```python
from build123d import *

# Parameters (mm, degrees)
SKETCH2_W           = 9.5
SKETCH2_H           = 9.5
BOSS_EXTRUDE1_DEPTH = 5
SKETCH3_R           = 4
BOSS_EXTRUDE2_DEPTH = 4
SKETCH4_R           = 3.25
BOSS_EXTRUDE3_DEPTH = 1.5
BOSS_EXTRUDE4_DEPTH = 7


with BuildPart() as part:
    # Sketch2 → Boss-Extrude1 (new body)
    with BuildSketch(Plane(origin=(0, 0, 0), x_dir=(1, 0, 0), z_dir=(0, 1, 0))):
        Rectangle(SKETCH2_W, SKETCH2_H)
    extrude(amount=BOSS_EXTRUDE1_DEPTH)

    # Sketch3 → Boss-Extrude2 (add)
    with BuildSketch(Plane(origin=(0, 5, 0), x_dir=(1, 0, 0), z_dir=(0, 1, 0))):
        with Locations(Location((0, 0, 0), (0, 0, 270))):
            Circle(SKETCH3_R)
    extrude(amount=BOSS_EXTRUDE2_DEPTH)

    # Sketch4 → Boss-Extrude3 (add)
    with BuildSketch(Plane(origin=(0, 9, 0), x_dir=(1, 0, 0), z_dir=(0, 1, 0))):
        with Locations(Location((0, 0, 0), (0, 0, 270))):
            Circle(SKETCH4_R)
    extrude(amount=BOSS_EXTRUDE3_DEPTH)

    # Sketch5 → Boss-Extrude4 (add)
    with BuildSketch(Plane.XZ):
        with BuildLine():
            Line((-2.5, -0.25), (2.5, -0.25))
            ThreePointArc((2.5, -0.25), (2.75, 0), (2.5, 0.25))
            Line((2.5, 0.25), (-2.5, 0.25))
            ThreePointArc((-2.5, 0.25), (-2.75, 0), (-2.5, -0.25))
        make_face()
    extrude(amount=BOSS_EXTRUDE4_DEPTH)


solid = part.part
```
Design review of the part built by this model. Coordinates are the model's own, in mm. A direction names the side the tool comes from. Give positions to 0.01 mm unless a question says otherwise; leave off trailing zeros. Order: outer loops, then holes, each group sorted by start corner. A loop starts at its lowest first (then second) coordinate and runs counter-clockwise, first axis right, second up. Notation, with made-up numbers: M 64.5,-29.75 L 68.5,-29.75 A31 cw 68.5,4.25 Z; hole C -18.75,44.5 d2. An arc over 180 degrees is marked long. One line per question, with ' | ' between items. Start each with the question number.
Q1. We need section C-C (y = 8.5). Write out the cut boundary in (x, z).
Q2. For pin 1 Ø5.5 at (x, y) = (-0.5, -3) entering from -Z; pin 2 Ø2.5 at (x, y) = (1, -2.5) entering from +Z; pin 3 Ø1.5 at (x, z) = (-0.5, -2) entering from -Y, all flat-tipped, find the tip position at first contact; note any pin that passes through.
Q3. Machinability: for faces 1 (the face through (-1.978, 9.74, -2.579)), 2 (the face through (0, 2, 4.75)), 3 (the face through (0, -3, -0.25)), 4 (the face through (0, -3, 0.25)), 5 (the face through (0, 2, -4.75)), which of the approach directions +Z, -Z, +X, -X, +Y, -Y give a long, thin tool a straight path to every point of the face, cutting with its end or side? Answer none if there is none.
Q4. We need section A-A (z = 0). Write out the cut boundary in (x, y).
Q5. For L1, parallel to Y at x = 3.25, z = -4; L2, parallel to Y at x = -3.25, z = -2; L3, parallel to Z at x = -1.25, y = -3, list the stretches that pass through material, from the lowest coordinate up. Write a range as [from, to].
Q6. We need section B-B (x = -3). Write out the cut boundary in (y, z), plus the area to 3 significant figures.
Q7. We need section D-D (x = 0). Write out the cut boundary in (y, z).
Returned:
1) outline: C 0,0 d8
2) pin 1: z = -0.25 | pin 2: z = 0.25 | pin 3: y = 0
3) face 1: +Y | face 2: +Z, +X, -X, +Y, -Y | face 3: -Z, +X, -X, -Y | face 4: +Z, +X, -X, -Y | face 5: -Z, +X, -X, +Y, -Y
4) outline: M -4.75,0 L -2.75,0 L -2.75,-7 L 2.75,-7 L 2.75,0 L 4.75,0 L 4.75,5 L 4,5 L 4,9 L 3.25,9 L 3.25,10.5 L -3.25,10.5 L -3.25,9 L -4,9 L -4,5 L -4.75,5 Z
5) L1: [0, 5] | L2: [0, 9] | L3: [-0.25, 0.25]
6) outline: M 0,-4.75 L 5,-4.75 L 5,-2.65 L 9,-2.65 L 9,-1.25 L 10.5,-1.25 L 10.5,1.25 L 9,1.25 L 9,2.65 L 5,2.65 L 5,4.75 L 0,4.75 Z | area: 72.4 mm2
7) outline: M -7,-0.25 L 0,-0.25 L 0,-4.75 L 5,-4.75 L 5,-4 L 9,-4 L 9,-3.25 L 10.5,-3.25 L 10.5,3.25 L 9,3.25 L 9,4 L 5,4 L 5,4.75 L 0,4.75 L 0,0.25 L -7,0.25 Z
